Source: CAD feature listing. Evaluate the final solid. Frame: model axes, mm. Round coordinates to 2 decimals unless told otherwise and drop trailing zeros. Order: outer loops, then holes, each group sorted by start corner. A loop starts at its lowest first (then second) coordinate and runs counter-clockwise, first axis right, second up. Notation, with made-up numbers: (19, 6.25) -> (25, 6.25) arc R21 cw to (25, 45.25) -> close; hole circle Ø3 at (-32.5, 52.5). An arc over 180 degrees is marked (long way). One line per item, written item: value. Start each with the question number.
1) Mould query, pull axis X, two halves, no side actions, for faces 1 (the face through (0, 5, 2.5)), 2 (the face through (21, 0, 0)), 3 (the face through (18.88, -17.01, 0.04)), 4 (the face through (-21, 0, 0)). Classes: pulls with the +X half, pulls with the -X half, needs draft (parallel to the pull), parting line crosses it, or undercut.
2) Section D-D (y = -1). Return the cut outline in (x, z), and give its area (3 significant figures).
3) Ray query, L1, parallel to Y at x = 17.4, z = 0.05; L2, parallel to Y at x = 0, z = 1.2; L3, parallel to Y at x = 16, z = -0.75. Return the intervals inside material, ascending.
4) Section B-B (y = -16.4). Return the cut outline in (x, z).
5) Section A-A (z = -1.9). Return the cut outline in (x, y).
6) Section C-C (x = 17.4). Return the cut outline in (y, z), and give its area (3 significant figures).
```python
from build123d import *

# Parameters (mm, degrees)
SKETCH1_W           = 42
SKETCH1_H           = 40
BOSS_EXTRUDE1_DEPTH = 2.5
SKETCH2_R           = 1.6
CUT_EXTRUDE1_DEPTH  = 30.427877939


with BuildPart() as part:
    # Sketch1 → Boss-Extrude1 (new, symmetric)
    with BuildSketch(Plane.XY):
        Rectangle(SKETCH1_W, SKETCH1_H)
    extrude(amount=BOSS_EXTRUDE1_DEPTH, both=True)

    # Sketch2 → Cut-Extrude1 (cut, through all)
    with BuildSketch(Plane.XY.offset(2.5)):
        with Locations((-17.4, 16.4)):
            Circle(SKETCH2_R)
        with Locations(Location((17.4, 16.4, 0), (0, 0, 180))):
            Circle(SKETCH2_R)
        with Locations((17.4, -16.4)):
            Circle(SKETCH2_R)
        with Locations(Location((-17.4, -16.4, 0), (0, 0, 180))):
            Circle(SKETCH2_R)
        Circle(SKETCH2_R)
    extrude(amount=-CUT_EXTRUDE1_DEPTH, mode=Mode.SUBTRACT)


solid = part.part
```
Findings:
1. face 1: needs draft
1. face 2: pulls with the +X half
1. face 3: undercut
1. face 4: pulls with the -X half
2. outline: (-21, -2.5) -> (-1.25, -2.5) -> (-1.25, 2.5) -> (-21, 2.5) -> close; (1.25, -2.5) -> (21, -2.5) -> (21, 2.5) -> (1.25, 2.5) -> close
2. area: 198 mm2
3. L1: -20 to -18, -14.8 to 14.8, 18 to 20
3. L2: -20 to -1.6, 1.6 to 20
3. L3: -20 to -17.17, -15.63 to 15.63, 17.17 to 20
4. outline: (-21, -2.5) -> (-19, -2.5) -> (-19, 2.5) -> (-21, 2.5) -> close; (-15.8, -2.5) -> (15.8, -2.5) -> (15.8, 2.5) -> (-15.8, 2.5) -> close; (19, -2.5) -> (21, -2.5) -> (21, 2.5) -> (19, 2.5) -> close
5. outline: (-21, -20) -> (21, -20) -> (21, 20) -> (-21, 20) -> close; hole circle Ø3.2 at (-17.4, -16.4); hole circle Ø3.2 at (-17.4, 16.4); hole circle Ø3.2 at (0, 0); hole circle Ø3.2 at (17.4, -16.4); hole circle Ø3.2 at (17.4, 16.4)
6. outline: (-20, -2.5) -> (-18, -2.5) -> (-18, 2.5) -> (-20, 2.5) -> close; (-14.8, -2.5) -> (14.8, -2.5) -> (14.8, 2.5) -> (-14.8, 2.5) -> close; (18, -2.5) -> (20, -2.5) -> (20, 2.5) -> (18, 2.5) -> close
6. area: 168 mm2
